For this review, use the dimensioned drawing (mm, ordinates from the lowest corner) and the shaded views. Coordinates: 2 decimals unless noted, no trailing zeros. Loops run counter-clockwise (first coordinate to the right, second up) from the corner with the lowest first, then second, coordinate; pieces in that order, holes last. Notation, with made-up numbers: (37.25, 15) - (59.25, 15) arc R22 cw to (59.25, 30) - close; hole circle Ø7 at (12.5, 17). An arc over 180 degrees is marked (long way). Answer in a Markdown table with one row per item. Add a question column.
(1) We need section A-A on z = 75.5. Write out the cut boundary in (x, y).
(2) For P1, Ø0.9, axis at x = 61, y = 1.5, coming from the +Z side; P2, Ø1.5, axis at y = 1, z = 60.5, coming from the -X side; P3, Ø0.9, axis at y = 1, z = 77.5, coming from the -X side; P4, Ø12, axis at x = 74.5, z = 67, coming from the -Y side, all flat-tipped, find the tip position at first contact; note any pin that passes through.
(3) We need section D-D on z = 55. Write out the cut boundary in (x, y).
(4) We need section C-C on z = 31.5. Write out the cut boundary in (x, y).
(5) For line 1 along X through (y, z) = (0.3, 41) (1 decimal); line 2 along X through (y, z) = (0.5, 26.5); line 3 along X through (y, z) = (2.3, 46.5) (1 decimal), list the stretches that pass through material, from the lowest coordinate up.
(6) We need section B-B on y = 1.35. Write out the cut boundary in (x, z) (1 decimal), plus the area to 3 significant figures.
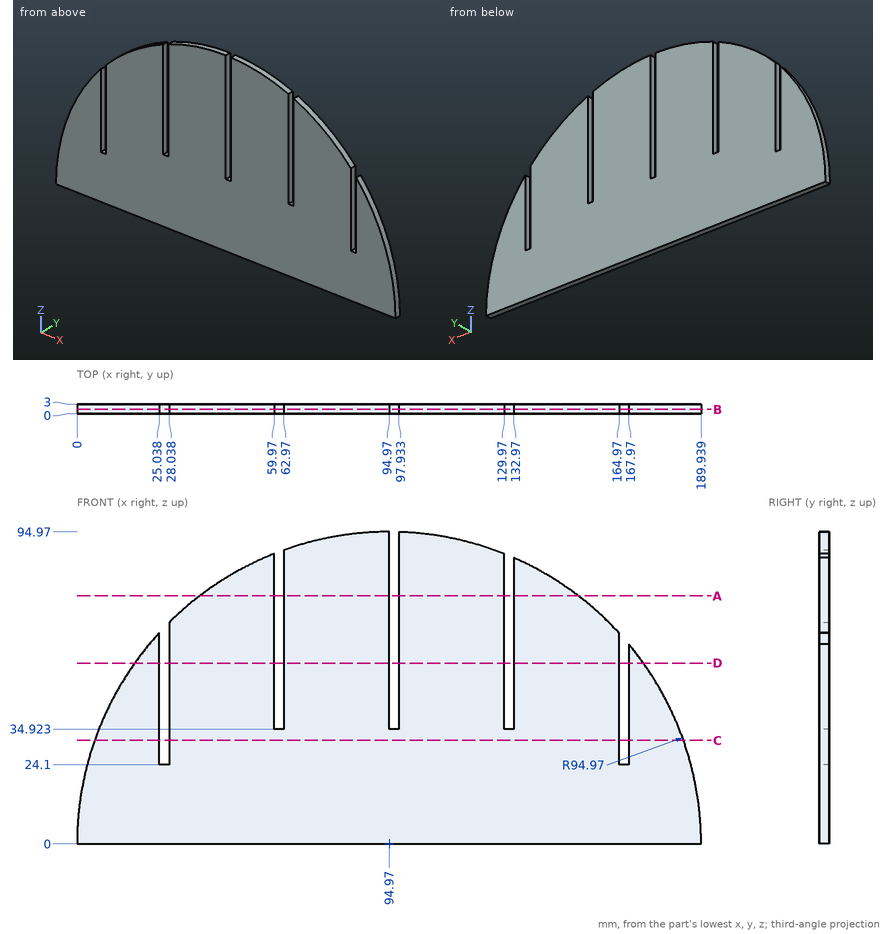
Outcome:
| question | item | result |
|---|---|---|
| 1 | outline | (37.36, 0) - (59.97, 0) - (59.97, 3) - (37.36, 3) - close; (62.97, 0) - (94.97, 0) - (94.97, 3) - (62.97, 3) - close; (97.93, 0) - (129.97, 0) - (129.97, 3) - (97.93, 3) - close; (132.97, 0) - (152.58, 0) - (152.58, 3) - (132.97, 3) - close |
| 2 | P1 | z = 34.92 |
| 2 | P2 | x = 21.15 |
| 2 | P3 | x = 39.45 |
| 2 | P4 | y = 0 |
| 3 | outline | (17.55, 0) - (25.04, 0) - (25.04, 3) - (17.55, 3) - close; (28.04, 0) - (59.97, 0) - (59.97, 3) - (28.04, 3) - close; (62.97, 0) - (94.97, 0) - (94.97, 3) - (62.97, 3) - close; (97.93, 0) - (129.97, 0) - (129.97, 3) - (97.93, 3) - close; (132.97, 0) - (164.97, 0) - (164.97, 3) - (132.97, 3) - close; (167.97, 0) - (172.39, 0) - (172.39, 3) - (167.97, 3) - close |
| 4 | outline | (5.38, 0) - (25.04, 0) - (25.04, 3) - (5.38, 3) - close; (28.04, 0) - (164.97, 0) - (164.97, 3) - (28.04, 3) - close; (167.97, 0) - (184.56, 0) - (184.56, 3) - (167.97, 3) - close |
| 5 | line 1 | 9.3 to 25, 28 to 60, 63 to 95, 97.9 to 130, 133 to 165, 168 to 180.6 |
| 5 | line 2 | 3.77 to 25.04, 28.04 to 164.97, 167.97 to 186.17 |
| 5 | line 3 | 12.2 to 25, 28 to 60, 63 to 95, 97.9 to 130, 133 to 165, 168 to 177.8 |
| 6 | outline | (0, 0) - (189.9, 0) arc R95 ccw to (168, 60.7) - (168, 24.1) - (165, 24.1) - (165, 64.2) arc R95 ccw to (133, 87) - (133, 34.9) - (130, 34.9) - (130, 88.3) arc R95 ccw to (97.9, 94.9) - (97.9, 34.9) - (95, 34.9) - (95, 95) arc R95 ccw to (63, 89.4) - (63, 34.9) - (60, 34.9) - (60, 88.3) arc R95 ccw to (28, 67.4) - (28, 24.1) - (25, 24.1) - (25, 64.3) arc R95 ccw to start |
| 6 | area | 13,400 mm² |
